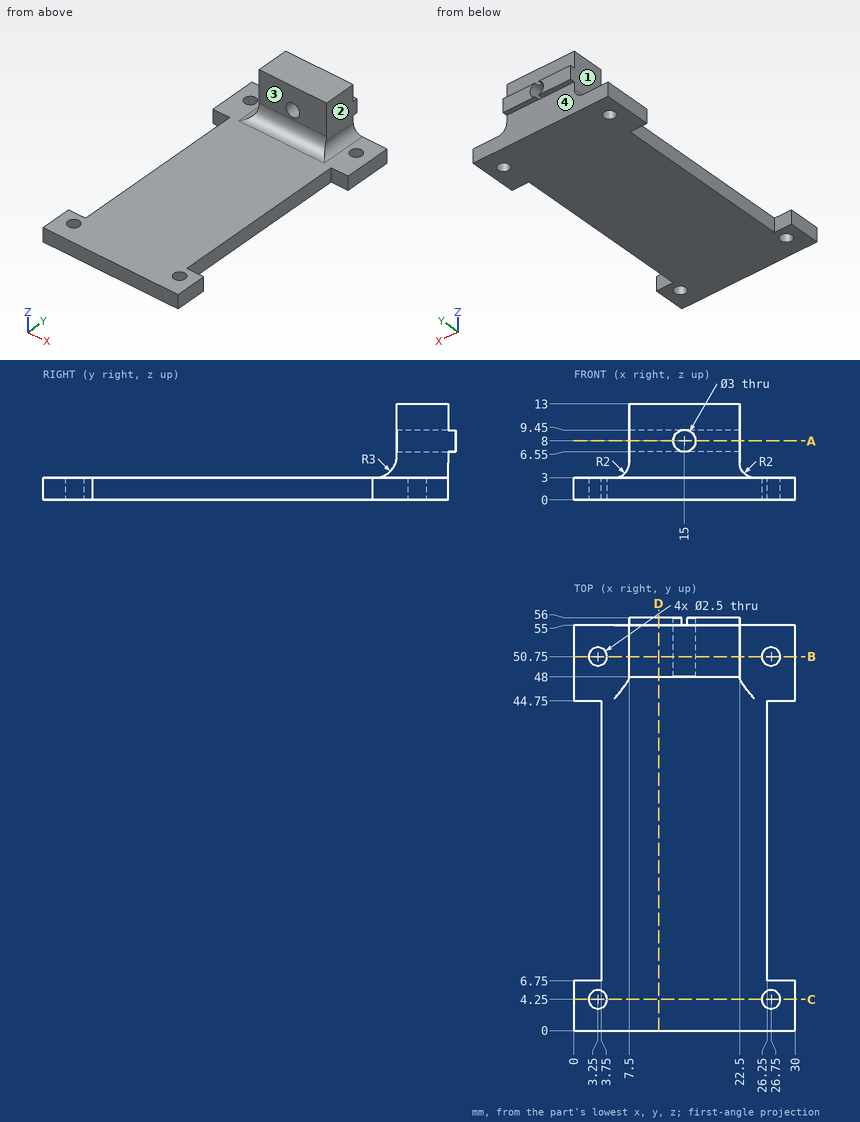
Part print with two shaded views. Sizes in mm from the minimum x, y, z corner. A direction names the side the tool comes from. Give positions to 0.01 mm unless a question says otherwise; leave off trailing zeros. Order: outer loops, then holes, each group sorted by start corner. A loop starts at its lowest first (then second) coordinate and runs counter-clockwise, first axis right, second up. Notation, with made-up numbers: M 29.5,-6 L 66.5,-6 A26 cw 66.5,29 Z; hole C 17.25,56.25 d6. An arc over 180 degrees is marked long. Put each result on its own line as item: value.
Item 1: Drop flat-ended pins along their axis: pin 1 Ø2 at (x, y) = (22, 25) entering from +Z; pin 2 Ø4 at (x, z) = (15, 8) entering from -Y; pin 3 Ø7 at (x, z) = (21, 2.5) entering from +Y; pin 4 Ø6 at (y, z) = (9.5, 8.5) entering from -X. Give the stop position or say it passes through.
Results are:
pin 1: z = 3
pin 2: y = 48
pin 3: y = 55
pin 4: through
Item 2: Cut at D-D on x = 11.5. Write the cut outline in (y, z), then the cut area to 3 significant figures.
Results are:
outline: M 0,0 L 55,0 L 55,6.55 L 56,6.55 L 56,9.45 L 55,9.45 L 55,13 L 48,13 L 48,6 A3 cw 45,3 L 0,3 Z
area: 240 mm2
Item 3: Wall check: probe 1 along Y at (x, z) = (3.25, 2.05); probe 2 along Z at (x, y) = (15, 50.25); probe 3 along Z at (x, y) = (9.5, 24.5). Give the ranges that are in metal, low to high.
Results are:
probe 1: 0 to 3, 5.5 to 6.75, 44.75 to 49.5, 52 to 55
probe 2: 0 to 6.5, 9.5 to 13
probe 3: 0 to 3
Item 4: Cut at B-B on y = 50.75. Write the cut outline in (x, z).
Results are:
outline: M 0,0 L 2,0 L 2,3 L 0,3 Z; M 4.5,0 L 25.5,0 L 25.5,3 L 24.5,3 A2 cw 22.5,5 L 22.5,13 L 7.5,13 L 7.5,5 A2 cw 5.5,3 L 4.5,3 Z; M 28,0 L 30,0 L 30,3 L 28,3 Z; hole C 15,8 d3
Item 5: Cut at A-A on z = 8. Write the cut outline in (x, y), then the cut area to 3 significant figures.
Results are:
outline: M 7.5,48 L 13.5,48 L 13.5,56 L 7.5,56 Z; M 16.5,48 L 22.5,48 L 22.5,56 L 16.5,56 Z
area: 96.0 mm2
Item 6: Which spindle directions (+Z, -Z, +X, -X, +Y, -Y) get a long thin tool onto all of the face, cutting with end or side? Do the marked faces 1, 2, 3 and 4. Say none if no direction does.
Results are:
face 1: +Z, -X, +Y, -Y
face 2: +Z, +X, +Y, -Y
face 3: +Z, +X, -X, -Y
face 4: -Z, +X, -X, +Y
Item 7: Cut at C-C on y = 4.25. Write the cut outline in (x, z), then the cut area to 3 significant figures.
Results are:
outline: M 0,0 L 2,0 L 2,3 L 0,3 Z; M 4.5,0 L 25.5,0 L 25.5,3 L 4.5,3 Z; M 28,0 L 30,0 L 30,3 L 28,3 Z
area: 75.0 mm2
